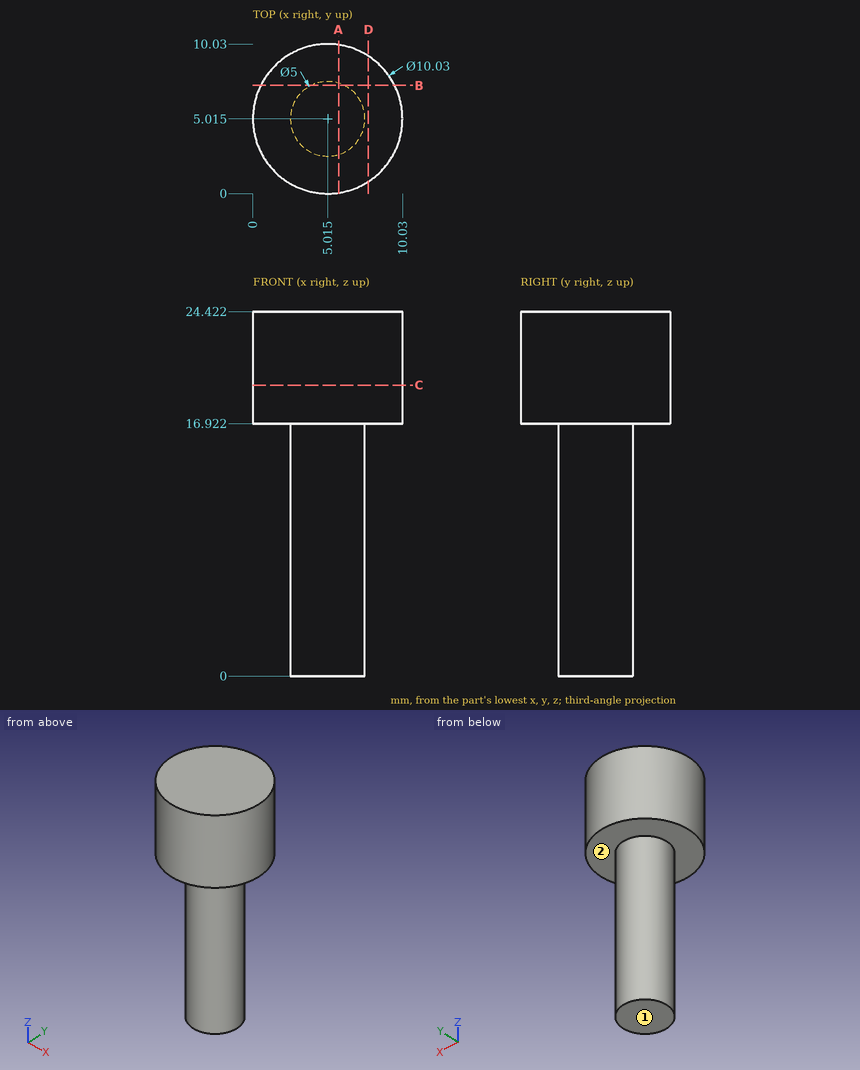
Part print with two shaded views. Sizes in mm from the minimum x, y, z corner. A direction names the side the tool comes from. Round coordinates to 2 decimals unless told otherwise and drop trailing zeros. Order: outer loops, then holes, each group sorted by start corner. A loop starts at its lowest first (then second) coordinate and runs counter-clockwise, first axis right, second up.
(1) Band-saw the part on A-A (x = 5.75). List the corners of the cut face in (y, z).
(2) Pin check, flat tips, straight feed: pin 1 (1 mm diameter, centred on x = 2, y = 7.5, fed in from -Z); pin 2 (2 mm diameter, centred on y = 4.5, z = 10.5, fed in from -X) (3 decimals); pin 3 (1 mm diameter, centred on x = 5, z = 12.5, fed in from -Y) (3 decimals). Stop position of each tip, or through.
(3) Band-saw the part on D-D (x = 7.75). List the corners of the cut face in (y, z).
(4) Band-saw the part on B-B (y = 7.25). List the corners of the cut face in (x, z), then the cut area to 3 significant figures.
(5) Drill centre lines: line 1 (Z direction, x = 2, y = 2.25); line 2 (Y direction, x = 7, z = 19.5); line 3 (X direction, y = 2.75, z = 6.75). Where is each one in solid material? Low to high.
(6) 3-axis set-ups, long thin cutter, end or side, ignore diameter. For the marked faces 1 and 2: which of +Z, -Z, +X, -X, +Y, -Y reach the whole face in a straight line?
(7) Band-saw the part on C-C (z = 19.5). List the corners of the cut face in (x, y) (3 decimals), then the cut area to 3 significant figures.
Verdict:
1. outline: (0.05, 16.92) - (2.63, 16.92) - (2.63, 0) - (7.4, 0) - (7.4, 16.92) - (9.98, 16.92) - (9.98, 24.42) - (0.05, 24.42) - close
2. pin 1: stops at z = 16.92
2. pin 2: stops at x = 2.515
2. pin 3: stops at y = 2.515
3. outline: (0.81, 16.92) - (9.22, 16.92) - (9.22, 24.42) - (0.81, 24.42) - close
4. outline: (0.53, 16.92) - (3.89, 16.92) - (3.89, 0) - (6.14, 0) - (6.14, 16.92) - (9.5, 16.92) - (9.5, 24.42) - (0.53, 24.42) - close
4. area: 105 mm2
5. line 1: z = 16.92 to 24.42
5. line 2: y = 0.41 to 9.62
5. line 3: x = 3.96 to 6.07
6. face 1: -Z, +X, -X, +Y, -Y
6. face 2: -Z
7. outline: circle Ø10.03 at (5.015, 5.015)
7. area: 79.0 mm2
